The listing builds one solid part. Answer for the finished solid, in the listing's coordinates (mm). Face numbers are marked on the shaded views. A direction names the side the tool comes from. Give positions to 0.01 mm unless a question says otherwise; leave off trailing zeros. Order: outer loops, then holes, each group sorted by start corner. A loop starts at its lowest first (then second) coordinate and runs counter-clockwise, first axis right, second up.
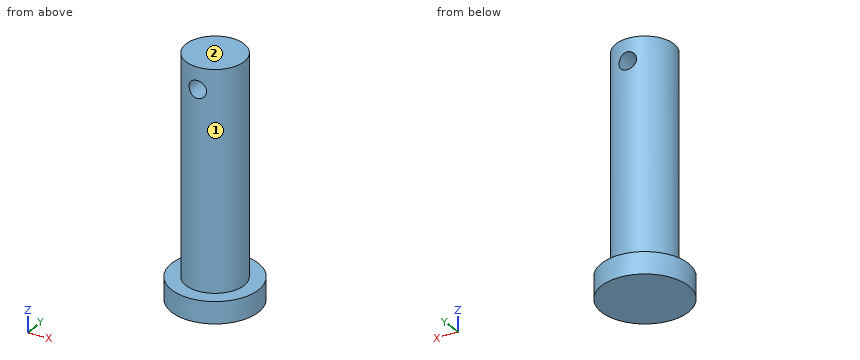
```python
from build123d import *

# Parameters (mm, degrees)
SKETCH2_R               = 6.7
BOSS_EXTRUDE1_DEPTH     = 55
SKETCH3_R               = 10
BOSS_EXTRUDE2_DEPTH     = 5
CUT_EXTRUDE1_DEPTH      = 10
CUT_EXTRUDE1_DEPTH_BACK = 15
SKETCH5_R               = 2


with BuildPart() as part:
    # Sketch2 → Boss-Extrude1 (new body)
    with BuildSketch(Plane.XY):
        Circle(SKETCH2_R)
    extrude(amount=BOSS_EXTRUDE1_DEPTH)

    # Sketch3 → Boss-Extrude2 (add)
    with BuildSketch(Plane(origin=(0, 0, 0), x_dir=(-1, 0, 0), z_dir=(0, 0, -1))):
        Circle(SKETCH3_R)
    extrude(amount=-BOSS_EXTRUDE2_DEPTH)

    # Sketch5 → Cut-Extrude1 (cut, two sides: drawn at the far end of the back side and taken through both)
    with BuildSketch(Plane(origin=(0, 0, 0), x_dir=(1, 0, 0), z_dir=(0, 1, 0)).offset(-CUT_EXTRUDE1_DEPTH_BACK)):
        with Locations(Location((0, -50, 0), (0, 0, 90))):
            Circle(SKETCH5_R)
    extrude(amount=CUT_EXTRUDE1_DEPTH + CUT_EXTRUDE1_DEPTH_BACK, mode=Mode.SUBTRACT)


solid = part.part
```
1) A tool of negligible diameter and unlimited length cuts with its end or side. For the marked faces 1 and 2, from which of +Z, -Z, +X, -X, +Y, -Y can it reach the whole face along a straight path? Write none if from no direction.
Geometry says:
face 1: +Z
face 2: +Z, +X, -X, +Y, -Y
2) Find section C-C (z = 50). Write down the section's boundary in (x, y), then the cut area to 3 significant figures.
Geometry says:
outline: (-2, -6.39) - (-2, 6.39) arc R6.7 ccw to start; (2, -6.39) arc R6.7 ccw to (2, 6.39) - close
area: 88.2 mm2
3) Find section A-A (x = 0). Write down the section's boundary in (y, z), then the cut area to 3 significant figures.
Geometry says:
outline: (-10, 0) - (10, 0) - (10, 5) - (6.7, 5) - (6.7, 48) - (-6.7, 48) - (-6.7, 5) - (-10, 5) - close; (-6.7, 52) - (6.7, 52) - (6.7, 55) - (-6.7, 55) - close
area: 716 mm2
4) Given P1, Ø10, axis at x = -1, z = 28.5, coming from the -Y side; P2, Ø2, axis at x = -6.5, y = 5, coming from the -Z side; P3, Ø6, axis at x = 4.5, z = 44, coming from the +Y side; P4, Ø1, axis at x = -0.5, z = 30.5, coming from the +Y side, each flat-ended and moving along its own axis, determine where each tip first touches the part or whether it passes through.
Geometry says:
P1: stops at y = -6.7
P2: stops at z = 0
P3: stops at y = 6.53
P4: stops at y = 6.7
5) Find section D-D (x = 3.25). Write down the section's boundary in (y, z), then the cut area to 3 significant figures.
Geometry says:
outline: (-9.46, 0) - (9.46, 0) - (9.46, 5) - (5.86, 5) - (5.86, 55) - (-5.86, 55) - (-5.86, 5) - (-9.46, 5) - close
area: 680 mm2
6) Find section B-B (y = 0). Write down the section's boundary in (x, z).
Geometry says:
outline: (-10, 0) - (10, 0) - (10, 5) - (6.7, 5) - (6.7, 55) - (-6.7, 55) - (-6.7, 5) - (-10, 5) - close; hole circle Ø4 at (0, 50)
7) Straight lines are drawn through the part: probe 1 along X at (y, z) = (2, 50); probe 2 along X at (y, z) = (-2.5, 50); probe 3 along Z at (x, y) = (7, 4.5). For each, find the intervals that lie inside material, in ascending order.
Geometry says:
probe 1: x = -6.39 to -2, 2 to 6.39
probe 2: x = -6.22 to -2, 2 to 6.22
probe 3: z = 0 to 5
